Autodesk Inventor part; units mm, degrees
ref_plane "Work Plane1" through (0, 1.5, 0) normal (0, 1, 0) x (1, 0, 0)
ref_plane "YZ Plane" through (0, 0, 0) normal (1, 0, 0) x (0, 1, 0)
ref_plane "XZ Plane" through (0, 0, 0) normal (0, 1, 0) x (-1, 0, 0)
sketch "Sketch1" plane through (0, 0, 0) normal (0, 1, 0) x (-1, 0, 0)
  line L0 (8.5, 8.5) -> (-8.5, 8.5)
  line L1 (-8.5, 8.5) -> (-8.5, -8.5)
  line L2 (-8.5, -8.5) -> (8.5, -8.5)
  line L3 (8.5, -8.5) -> (8.5, 8.5)
  line L4 (8.5, 8.5) -> (-8.5, -8.5) construction
  line L5 (-8.5, 8.5) -> (8.5, -8.5) construction
  line L6 (6, 6) -> (-6, 6)
  line L7 (-6, 6) -> (-6, -6)
  line L8 (-6, -6) -> (6, -6)
  line L9 (6, -6) -> (6, 6)
  line L10 (6, 6) -> (-6, -6) construction
  line L11 (-6, 6) -> (6, -6) construction
  circle A0 centre (6, 6) radius 1.5
  line L12 (6, 0) -> (4.5, 0)
  line L13 (0, 6) -> (0, 3.3641)
  circle A1 centre (6, -6) radius 1.5
  circle A2 centre (-6, 6) radius 1.5
  circle A3 centre (-6, -6) radius 1.5
  circle A4 centre (0, 0) radius 4.5
  dimension "d0" = 17
  dimension "d1" = 17
  dimension "d2" = 12
  dimension "d3" = 12
  dimension "d4" = 3
  dimension "d5" = 9
extrude "Extrusion1" add sketch "Sketch1" along normal blind 1.5 contours L3 L2 L1 L0 | L13 A4 L12 L9 A1 L8 A3 L7 A2 L6 | L6 A0 L9 L12 A4 L13 | A4
ref_plane "Work Plane1" through (0, 1.5, 0) normal (0, 1, 0) x (1, 0, 0)
sketch "Sketch2" plane through (0, 1.5, 0) normal (0, 1, 0) x (1, 0, 0)
  circle A0 centre (0, 0) radius 4.5
  dimension "d9" = 9
extrude "Extrusion2" add sketch "Sketch2" along normal blind 18
properties part number "BNC connector"
Source: CAD feature listing. Evaluate the final solid. Frame: model axes, mm. A direction names the side the tool comes from. Give positions to 0.01 mm unless a question says otherwise; leave off trailing zeros. Loops run counter-clockwise (first coordinate to the right, second up) from the corner with the lowest first, then second, coordinate; pieces in that order, holes last. Notation, with made-up numbers: (41, -38) -> (92, -38) arc R9 ccw to (92, -28) -> close; hole circle Ø6 at (82, 8). An arc over 180 degrees is marked (long way). Use a Markdown table: item, result. Add a question column.
1) Section query A-A, the plane x = 6. Return the cut outline in (y, z), then the cut area to 3 significant figures.
2) Section query C-C, the plane z = 0. Return the cut outline in (x, y).
3) Line query: line 1 along X through (y, z) = (0.5, 6); line 2 along Y through (x, z) = (-5.75, 0.75). Output: solid intervals per line, ascending. Write a range as [from, to].
4) Reachability of faces 4 (the face through (0, 1, 8.5)), 5 (the face through (4, 1.5, 4)) from +Z, -Z, +X, -X, +Y, -Y: full face, straight path, thin tool, end or side. Return the list, or none.
5) First-contact query: pin 1 (3 mm diameter, centred on y = 14.5, z = 1, fed in from +X); pin 2 (8 mm diameter, centred on y = 9, z = 5.5, fed in from +X); pin 3 (1 mm diameter, centred on y = 6.5, z = -4.5, fed in from -X); pin 4 (1.8 mm diameter, centred on x = -6, z = -6, fed in from +Y). Flat tips, straight axial feed; report the tip coordinate or a pass-through.
6) Pull-direction query (Z, two-part tool) for faces 1 (the face through (-0.59, 10.37, 4.46)), 2 (the face through (7.2, 0.7, 6.9)), 3 (the face through (0, 19.5, 0)); classes: +Z half, -Z half, draft (parallel to the pull), parting line (faces both ways), or undercut.
7) Section query B-B, the plane z = 6. Return the cut outline in (x, y).
8) Section query D-D, the plane x = 0. Return the cut outline in (y, z).
Numbers:
| question | item | result |
|---|---|---|
| 1 | outline | (0, -8.5) -> (1.5, -8.5) -> (1.5, -7.5) -> (0, -7.5) -> close; (0, -4.5) -> (1.5, -4.5) -> (1.5, 4.5) -> (0, 4.5) -> close; (0, 7.5) -> (1.5, 7.5) -> (1.5, 8.5) -> (0, 8.5) -> close |
| 1 | area | 16.5 mm2 |
| 2 | outline | (-8.5, 0) -> (8.5, 0) -> (8.5, 1.5) -> (4.5, 1.5) -> (4.5, 19.5) -> (-4.5, 19.5) -> (-4.5, 1.5) -> (-8.5, 1.5) -> close |
| 3 | line 1 | x = [-8.5, -7.5], [-4.5, 4.5], [7.5, 8.5] |
| 3 | line 2 | y = [0, 1.5] |
| 4 | face 4 | +Z, +X, -X, +Y, -Y |
| 4 | face 5 | +Y |
| 5 | pin 1 | stops at x = 4.5 |
| 5 | pin 2 | stops at x = 4.24 |
| 5 | pin 3 | stops at x = -2.06 |
| 5 | pin 4 | passes through |
| 6 | face 1 | parting line |
| 6 | face 2 | undercut |
| 6 | face 3 | draft |
| 7 | outline | (-8.5, 0) -> (-7.5, 0) -> (-7.5, 1.5) -> (-8.5, 1.5) -> close; (-4.5, 0) -> (4.5, 0) -> (4.5, 1.5) -> (-4.5, 1.5) -> close; (7.5, 0) -> (8.5, 0) -> (8.5, 1.5) -> (7.5, 1.5) -> close |
| 8 | outline | (0, -8.5) -> (1.5, -8.5) -> (1.5, -4.5) -> (19.5, -4.5) -> (19.5, 4.5) -> (1.5, 4.5) -> (1.5, 8.5) -> (0, 8.5) -> close |
